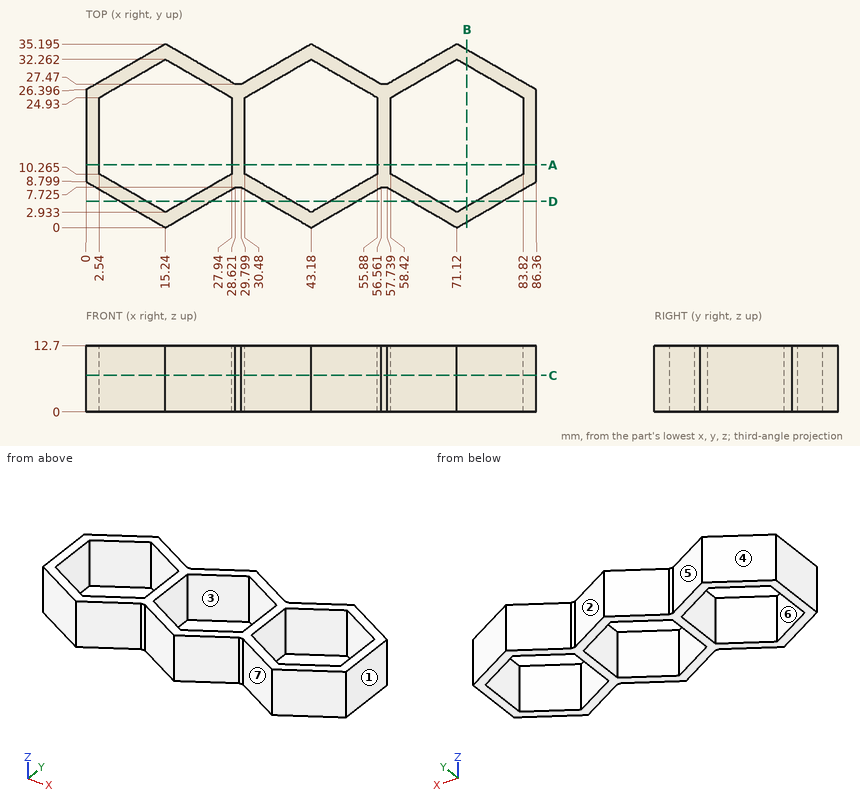
Input: dimensioned drawing with shaded views. Units: mm. Origin: part minimum x, y, z. A direction names the side the tool comes from. Round coordinates to 2 decimals unless told otherwise and drop trailing zeros. Write each loop counter-clockwise with the first axis right and the second up, starting at its lowest first coordinate (ties: lowest second). Pieces come first, ordered by that corner, then holes. Notation, with made-up numbers: (-26, 72.25) - (-13, 72.25) arc R14 cw to (-13, 94.25) - close; hole circle Ø9 at (46, -3). An arc over 180 degrees is marked (long way). Write item = value, one per line.
(1) Section query B-B on x = 73. Output: boundary loops of the cut face in (y, z) (1 decimal).
Geometry check:
outline = (1.1, 0) - (4, 0) - (4, 12.7) - (1.1, 12.7) - close; (31.2, 0) - (34.1, 0) - (34.1, 12.7) - (31.2, 12.7) - close
(2) Section query A-A on y = 12. Output: boundary loops of the cut face in (x, z), then the cut area to 3 significant figures.
Geometry check:
outline = (0, 0) - (2.54, 0) - (2.54, 12.7) - (0, 12.7) - close; (27.94, 0) - (30.48, 0) - (30.48, 12.7) - (27.94, 12.7) - close; (55.88, 0) - (58.42, 0) - (58.42, 12.7) - (55.88, 12.7) - close; (83.82, 0) - (86.36, 0) - (86.36, 12.7) - (83.82, 12.7) - close
area = 129 mm^2
(3) Access query for the marked faces 5, 6 and 7. Directions: +Z, -Z, +X, -X, +Y, -Y. A direction counts if a zero-diameter tool reaches every point of the face in a straight line with its end or side. Return the directions, or none.
Geometry check:
face_5 = +Z, -Z, +Y
face_6 = +Z, -Z
face_7 = +Z, -Z, -Y
(4) Contact query for flat-ended pins moving along their axis: pin 1 Ø1.5 at (x, z) = (74, 10.5) entering from +Y (1 decimal); pin 2 Ø1.3 at (x, z) = (57, 8) entering from +Y; pin 3 Ø6.5 at (y, z) = (15, 5.5) entering from -X; pin 4 Ø4 at (x, z) = (10.5, 6) entering from -Y. Output: stop coordinate, or through.
Geometry check:
pin_1 = 34
pin_2 = 27.59
pin_3 = 0
pin_4 = 1.58
(5) Section query C-C on z = 7. State how many separate pieces and enclosed holes the cut face has.
Geometry check:
separate_pieces = 1
enclosed_holes = 3
(6) Pull-direction query (X, two-part tool) for the marked faces 1, 2, 3 and 4; classes: +X half, -X half, draft (parallel to the pull), parting line (faces both ways), or undercut.
Geometry check:
face_1 = +X half
face_2 = undercut
face_3 = undercut
face_4 = -X half
(7) Section query D-D on y = 5. Output: boundary loops of the cut face in (x, z), then the cut area to 3 significant figures.
Geometry check:
outline = (6.58, 0) - (11.66, 0) - (11.66, 12.7) - (6.58, 12.7) - close; (18.82, 0) - (23.9, 0) - (23.9, 12.7) - (18.82, 12.7) - close; (34.52, 0) - (39.6, 0) - (39.6, 12.7) - (34.52, 12.7) - close; (46.76, 0) - (51.84, 0) - (51.84, 12.7) - (46.76, 12.7) - close; (62.46, 0) - (67.54, 0) - (67.54, 12.7) - (62.46, 12.7) - close; (74.7, 0) - (79.78, 0) - (79.78, 12.7) - (74.7, 12.7) - close
area = 387 mm^2
(8) Material intervals for probe 1 along X at (y, z) = (17, 8.5); probe 2 along X at (y, z) = (29.5, 4.5) (1 decimal); probe 3 along X at (y, z) = (25, 8.25) (1 decimal), sorted ascending.
Geometry check:
probe_1 = 0 to 2.54, 27.94 to 30.48, 55.88 to 58.42, 83.82 to 86.36
probe_2 = 5.4 to 10.5, 20 to 25.1, 33.3 to 38.4, 48 to 53, 61.3 to 66.3, 75.9 to 81
probe_3 = 0 to 2.7, 27.8 to 30.6, 55.8 to 58.5, 83.7 to 86.4
